Verification items for the finished model (mm, model axes). Face numbers are marked on the shaded views. Coordinates: 2 decimals unless noted, no trailing zeros. Order: outer loops, then holes, each group sorted by start corner. A loop starts at its lowest first (then second) coordinate and runs counter-clockwise, first axis right, second up. Notation, with made-up numbers: (-20.5, 65.5) -> (2.5, 65.5) arc R17 cw to (2.5, 98.5) -> close; hole circle Ø8 at (31, 39). An arc over 180 degrees is marked (long way). Write each question's results on one line, items separated by ' | '. Start each with the question number.
(1) Go/stop test with flat-tipped pins: pin 1 (2 mm diameter, centred on x = 43.5, z = 4, fed in from +Y); pin 2 (4 mm diameter, centred on x = 42.5, z = -4.5, fed in from +Y); pin 3 (5 mm diameter, centred on x = 35, z = 5.5, fed in from -Y). Record where each tip stops, or that it passes through.
(2) Draft check along Z on the marked faces 1 and 2. Enter one of: +Z half, -Z half, draft (parallel to the pull), parting line (faces both ways), or undercut.
(3) Thickness scan on probe 1 along X at (y, z) = (2.25, 4.5); probe 2 along Y at (x, z) = (12.5, 3); probe 3 along X at (y, z) = (-3, 2.5). Record the ranges inside material, lowest first. Write a range as [from, to].
(4) Cross-section at A-A on x = 11. Enter the section's corners in (y, z).
```python
from build123d import *

# Parameters (mm, degrees)
CHAMFER_1_SIZE = 0.25
SKETCH_2_W     = 1.2
SKETCH_2_H     = 0.35
FILLET_1_R     = 5
CHAMFER_2_SIZE = 1


with BuildPart() as part:
    # Эскиз1 → Повернуть1 (revolve)
    with BuildSketch(Plane.XY, mode=Mode.PRIVATE) as revolve_1_sk:
        Polygon((0, 0), (0, 7.5), (4, 7.5), (4, 5.1), (62, 5.1), (62, 0), align=None)
    revolve(revolve_1_sk.sketch.rotate(Axis((0, 0, 0), (1, 0, 0)), 90), axis=Axis((0, 0, 0), (1, 0, 0)))

    # Фаска1
    chamfer_1_edges = [part.edges().sort_by_distance(p)[0] for p in [
        (4, 0, -7.5),
    ]]
    chamfer(chamfer_1_edges, length=CHAMFER_1_SIZE)

    # Эскиз2 → Вырез-Повернуть1 (revolve, cut)
    with BuildSketch(Plane.XY, mode=Mode.PRIVATE) as cut_revolve_1_sk:
        with Locations((59.6, 4.925)):
            Rectangle(SKETCH_2_W, SKETCH_2_H)
    revolve(cut_revolve_1_sk.sketch.rotate(Axis((0, 0, 0), (1, 0, 0)), 90), axis=Axis((0, 0, 0), (1, 0, 0)), mode=Mode.SUBTRACT)

    # Скругление1
    # the kernel refuses this fillet: 5 mm, written as the material it takes off along each edge
    with BuildSketch(Plane(origin=(0, 0, 0), x_dir=(0, 0, 1), z_dir=(0, 1, 0))) as fillet_1_piece_1:
        with BuildLine():
            CenterArc((2.658770817, 5), FILLET_1_R, 270, 75.522487814)
            Line((2.658770817, 0), (2.658770817, -0.1))
            Line((2.658770817, -0.1), (7.5, -0.1))
            Line((7.5, -0.1), (7.6, 0))
            ThreePointArc((7.6, 0), (7.6, 1.875), (7.596824584, 3.725))
            Line((7.596824584, 3.725), (7.5, 3.75))
        make_face()
    revolve(axis=Axis((0, 0, 0), (1, 0, 0)), mode=Mode.SUBTRACT)

    # Фаска2
    chamfer_2_edges = [part.edges().sort_by_distance(p)[0] for p in [
        (62, 0, -5.1),
    ]]
    chamfer(chamfer_2_edges, length=CHAMFER_2_SIZE)


solid = part.part
```
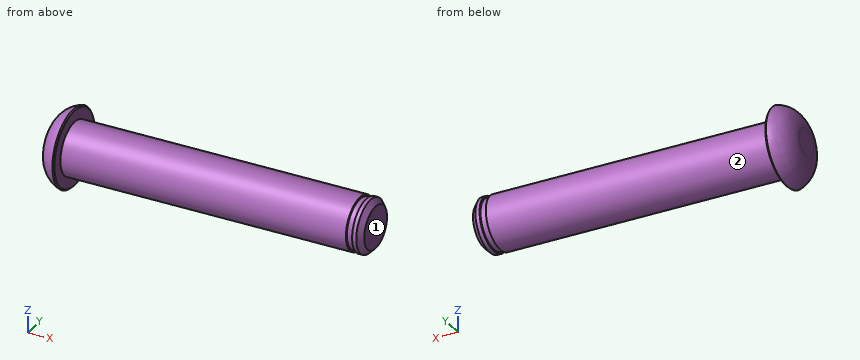
Results are:
1) pin 1: stops at y = 4.12 | pin 2: stops at y = 4.45 | pin 3: stops at y = -4.12
2) face 1: draft | face 2: parting line
3) probe 1: x = [0.6, 59], [60.2, 61.07] | probe 2: y = [-4.12, 4.12] | probe 3: x = [0.16, 62]
4) outline: circle Ø10.2 at (0, 0)
